Here's the drawing with two shaded views (mm, measured from the low corner). I have some questions. Give positions to 0.01 mm unless a question says otherwise; leave off trailing zeros. Write each loop counter-clockwise with the first axis right and the second up, starting at its lowest first coordinate (ties: lowest second). Pieces come first, ordered by that corner, then holes.
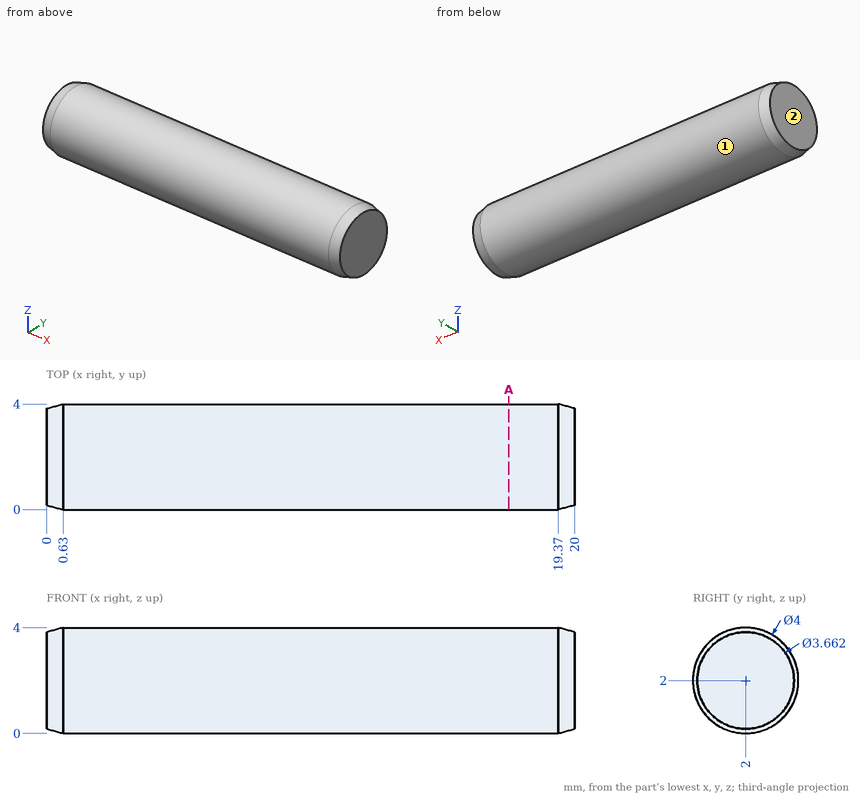
(1) If I drill on L1, parallel to Z at x = 12.75, y = 1.9; L2, parallel to Y at x = 8, z = 2.35; L3, parallel to Z at x = 7.5, y = 3.75 (1 decimal), over which ranges is the centre line in solid material (lowest first)?
Returned:
L1: z = 0 to 4
L2: y = 0.03 to 3.97
L3: z = 1 to 3
(2) Will these pins go through, and if not, where does the flat tip stop? P1, Ø1, axis at x = 16, z = 1.5, coming from the -Y side; P2, Ø1, axis at x = 11, y = 3.5, coming from the -Z side.
Returned:
P1: stops at y = 0
P2: stops at z = 0.27
(3) Imagine slicing it at A-A, the plane x = 17.5. Write out the boundary of the cut face in (y, z).
Returned:
outline: circle Ø4 at (2, 2)
(4) If we mould it in two halves opening along Z, with no side actions, what happens to the marked faces 1 and 2? For each: +Z half, -Z half, draft (parallel to the pull), parting line (faces both ways), or undercut.
Returned:
face 1: parting line
face 2: draft
